Verification items for the finished model (mm, model axes). A direction names the side the tool comes from. Round coordinates to 2 decimals unless told otherwise and drop trailing zeros. Loops run counter-clockwise (first coordinate to the right, second up) from the corner with the lowest first, then second, coordinate; pieces in that order, holes last. Notation, with made-up numbers: (38.5, 63) -> (54.5, 63) arc R11 ccw to (54.5, 73) -> close; hole circle Ø11 at (-16, -15.5). An arc over 180 degrees is marked (long way). Write item = value, one per line.
```python
from build123d import *

# Parameters (mm, degrees)
F0_W     = 25.4
F0_H     = 3.175
F1_DEPTH = 584.2
F2_R     = 2.1844
F3_DEPTH = 25.4
F4_R     = 2.1844
F5_DEPTH = 25.4


with BuildPart() as f1:
    # F0 (on Top) → F1 (new body)
    with BuildSketch(Plane.XY):
        with Locations((12.7, -1.5875)):
            Rectangle(F0_W, F0_H)
        Polygon((207.4032145214, -45.5008036304), (25.4, 0), (25.4, -3.175), (194.7032145214, -45.5008036304), align=None)
        with Locations((241.3, -52.3875)):
            Rectangle(F0_W, F0_H)
        Polygon((228.6, -50.8), (212.4832145214, -46.7708036304), (199.7832145214, -46.7708036304), (228.6, -53.975), align=None)
        Polygon((212.4832145214, -46.7708036304), (207.4032145214, -45.5008036304), (194.7032145214, -45.5008036304), (199.7832145214, -46.7708036304), align=None)
    extrude(amount=F1_DEPTH)

    # F2 (on face) → F3 (cut)
    with BuildSketch(Plane.XZ.offset(3.175)):
        with Locations((12.7, 121.92)):
            Circle(F2_R)
        with Locations((12.7, 292.1)):
            Circle(F2_R)
        with Locations((12.7, 462.28)):
            Circle(F2_R)
    extrude(amount=-F3_DEPTH, mode=Mode.SUBTRACT)

    # F4 (on face) → F5 (cut)
    with BuildSketch(Plane.XZ.offset(53.975)):
        with Locations((241.3, 292.1)):
            Circle(F4_R)
        with Locations((241.3, 462.28)):
            Circle(F4_R)
        with Locations((241.3, 121.92)):
            Circle(F4_R)
    extrude(amount=-F5_DEPTH, mode=Mode.SUBTRACT)


solid = f1.part
```
(1) Sectioned sample at A-A, the plane z = 68.5. Record the cut outline in (x, y) (3 decimals), and give its area (3 significant figures).
Filled sheet:
outline = (0, -3.175) -> (25.4, -3.175) -> (228.6, -53.975) -> (254, -53.975) -> (254, -50.8) -> (228.6, -50.8) -> (25.4, 0) -> (0, 0) -> close
area = 806 mm2
(2) Sectioned sample at B-B, the plane y = -35. Record the cut outline in (x, z), and give its area (3 significant figures).
Filled sheet:
outline = (152.7, 0) -> (165.4, 0) -> (165.4, 584.2) -> (152.7, 584.2) -> close
area = 7,420 mm2
(3) Set-up check for faces 1 (the face through (13, -3.175, 288)), 2 (the face through (241, -50.8, 288)), 3 (the face through (241, -53.975, 288)): record each of +Z, -Z, +X, -X, +Y, -Y from which the full face is reachable in a straight line by a thin tool's end or side.
Filled sheet:
face_1 = +Z, -Z, -X, -Y
face_2 = +Z, -Z, +X, +Y
face_3 = +Z, -Z, +X, -X, -Y
(4) Go/stop test with flat-tipped pins: pin 1 Ø4 at (x, z) = (241.3, 462.28) entering from -Y; pin 2 Ø5 at (x, z) = (156, 166.5) entering from -Y; pin 3 Ø20.5 at (x, z) = (242.5, 319.5) entering from +Y; pin 4 Ø8 at (x, z) = (189, 315) entering from +Y. Record where each tip stops, or that it passes through.
Filled sheet:
pin_1 = through
pin_2 = -36.45
pin_3 = -50.8
pin_4 = -39.9
(5) Material ranges on probe 1 along Z at (x, y) = (241.3, -52.75); probe 2 along Y at (x, z) = (22.5, 530.5) (3 decimals); probe 3 along Y at (x, z) = (153.5, 488) (3 decimals), recorded low to high. Write a range as from..to.
Filled sheet:
probe_1 = 0..119.74, 124.1..289.92, 294.28..460.1, 464.46..584.2
probe_2 = -3.175..0
probe_3 = -35.2..-32.025
(6) Sectioned sample at C-C, the plane x = 83.5. Record the cut outline in (y, z) (3 decimals).
Filled sheet:
outline = (-17.7, 0) -> (-14.525, 0) -> (-14.525, 584.2) -> (-17.7, 584.2) -> close
